Here's how the part is built. I have some questions about the finished solid (model axes, mm). Face numbers are marked on the shaded views. A direction names the side the tool comes from. Round coordinates to 2 decimals unless told otherwise and drop trailing zeros. Order: outer loops, then holes, each group sorted by start corner. A loop starts at its lowest first (then second) coordinate and runs counter-clockwise, first axis right, second up. Notation, with made-up numbers: (-8, 23) -> (12, 23) arc R23 ccw to (12, 49) -> close; hole circle Ø4 at (41, 78.5). An arc over 180 degrees is marked (long way). Answer in a Markdown table with one row per item.
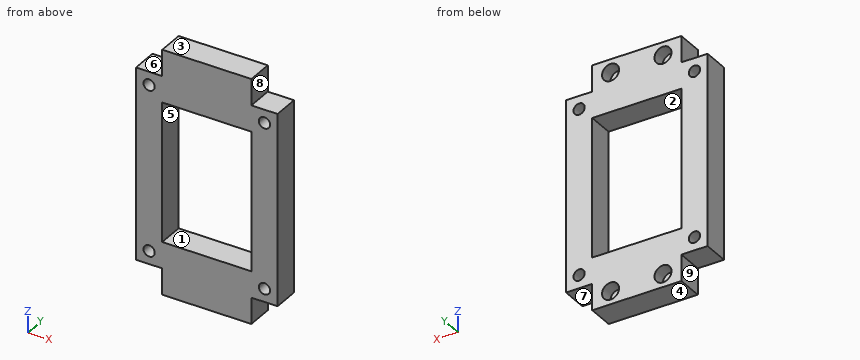
Autodesk Inventor part; units mm, degrees
ref_plane "YZ Plane" through (0, 0, 0) normal (1, 0, 0) x (0, 1, 0)
ref_plane "XZ Plane" through (0, 0, 0) normal (0, 1, 0) x (-1, 0, 0)
ref_plane "XY Plane" through (0, 0, 0) normal (0, 0, 1) x (1, 0, 0)
sketch "Sketch1" plane through (0, 0, 0) normal (0, 1, 0) x (-1, 0, 0)
  line L0 (0, 0) -> (10, 0)
  line L1 (10, 0) -> (10, 10)
  line L2 (10, 10) -> (44, 10)
  line L3 (44, 10) -> (44, 0)
  line L4 (44, 0) -> (54, 0)
  line L5 (54, 0) -> (54, -73)
  line L6 (54, -73) -> (44, -73)
  line L7 (44, -73) -> (44, -83)
  line L8 (44, -83) -> (10, -83)
  line L9 (10, -83) -> (10, -73)
  line L10 (10, -73) -> (0, -73)
  line L11 (0, -73) -> (0, 0)
  dimension "d9" = 73
  dimension "d10" = 54
  dimension "thickness" = 10
  dimension "t" = 10
  dimension "d13" = 10
  dimension "d14" = 10
  dimension "d15" = 10
  dimension "d16" = 10
  dimension "d17" = 10
extrude "Extrusion1" add sketch "Sketch1" along normal blind 10
hole "Hole1" at (-49, 10, -5) direction (0, -1, 0) diameter 4.3 end through all
hole "Hole2" at (-5, 10, -5) direction (0, -1, 0) diameter 4.3 end through all
hole "Hole3" at (-5, 10, -68) direction (0, -1, 0) diameter 4.3 end through all
hole "Hole4" at (-49, 10, -68) direction (0, -1, 0) diameter 4.3 end through all
sketch "Sketch2" plane through (0, 10, 0) normal (0, 1, 0) x (1, 0, 0)
  circle A0 centre (-37, -5) radius 3.25
  circle A1 centre (-17, -5) radius 3.25
  circle A2 centre (-37, 78) radius 3.25
  circle A3 centre (-17, 78) radius 3.25
  line L0 (-44, -10) -> (-10, -10)
  line L1 (-10, 83) -> (-44, 83)
  line L2 (-44, 0) -> (-44, -10)
  line L3 (-10, -10) -> (-10, 0)
  line L4 (-10, 73) -> (-10, 83)
  line L5 (-44, 83) -> (-44, 73)
  point P0 (0, 0)
  dimension "d56" = 6.5
  dimension "d57" = 6.5
  dimension "d58" = 6.5
  dimension "d59" = 6.5
  dimension "d60" = 5
  dimension "d61" = 5
  dimension "d62" = 5
  dimension "d63" = 5
  dimension "d64" = 7
  dimension "d65" = 7
  dimension "d66" = 7
  dimension "d67" = 7
extrude "Extrusion2" cut sketch "Sketch2" against normal blind 5
sketch "Sketch3" plane through (0, 0, 0) normal (0, -1, 0) x (1, 0, 0)
  line L0 (-44, -10) -> (-10, -10)
  line L1 (-10, -10) -> (-10, -63)
  line L2 (-10, -63) -> (-44, -63)
  line L3 (-44, -63) -> (-44, -10)
  line L4 (-10, 10) -> (-44, 10)
  line L5 (-44, -83) -> (-10, -83)
  line L6 (0, -73) -> (0, 0)
  line L7 (-54, 0) -> (-54, -73)
  dimension "d70" = 20
  dimension "d71" = 20
  dimension "d72" = 10
  dimension "d73" = 10
extrude "Extrusion3" cut sketch "Sketch3" against normal blind 10
equation "\"thickness\" = t"
equation "\"d13\" = t"
equation "\"d14\" = t"
equation "\"d15\" = t"
equation "\"d16\" = t"
equation "\"d17\" = t"
equation "\"d18\" = t"
properties part number "backFrame"
1. For the marked faces 5, 6, 7, 8 and 9, which set-ups out of +Z, -Z, +X, -X, +Y, -Y let a thin tool reach every point of the face, with its end or its side?
Numbers:
| item | result |
|---|---|
| face 5 | +Y, -Y |
| face 6 | +Z, -X, +Y, -Y |
| face 7 | -Z, +X, +Y, -Y |
| face 8 | +Z, +X, +Y, -Y |
| face 9 | -Z, -X, +Y, -Y |
2. Suppose I cut it at C-C on y = 8. State how many separate pieces and enclosed holes the cut face has, then the cut area to 3 significant figures.
Numbers:
| item | result |
|---|---|
| separate pieces | 1 |
| enclosed holes | 9 |
| area | 2,630 mm2 |
3. Suppose I cut it at D-D on z = -25. Write out the boundary of the cut face in (x, y), then the cut area to 3 significant figures.
Numbers:
| item | result |
|---|---|
| outline | (-54, 0) -> (-44, 0) -> (-44, 10) -> (-54, 10) -> close; (-10, 0) -> (0, 0) -> (0, 10) -> (-10, 10) -> close |
| area | 200 mm2 |
4. For pin 1 Ø5 at (x, y) = (-4.5, 7) entering from -Z; pin 2 Ø3 at (y, z) = (3, -79.5) entering from +X; pin 3 Ø3 at (x, z) = (-37.5, 5) entering from +Y, each with a flat end and sliding along its axis, tell me the tip position at first contact or that it passes through.
Numbers:
| item | result |
|---|---|
| pin 1 | stops at z = -73 |
| pin 2 | stops at x = -10 |
| pin 3 | stops at y = 5 |
5. We'd pull the mould along Z, two halves only. Please class the marked faces 1, 2, 3 and 4: released by +Z, released by -Z, zero draft, split by the parting line, or undercut.
Numbers:
| item | result |
|---|---|
| face 1 | undercut |
| face 2 | undercut |
| face 3 | released by +Z |
| face 4 | released by -Z |
6. Suppose I cut it at A-A on x = -28.5. Write out the boundary of the cut face in (y, z), then the cut area to 3 significant figures.
Numbers:
| item | result |
|---|---|
| outline | (0, -83) -> (10, -83) -> (10, -63) -> (0, -63) -> close; (0, -10) -> (10, -10) -> (10, 10) -> (0, 10) -> close |
| area | 400 mm2 |
7. Suppose I cut it at B-B on z = -5. Write out the boundary of the cut face in (x, y), then the cut area to 3 significant figures.
Numbers:
| item | result |
|---|---|
| outline | (-54, 0) -> (-51.15, 0) -> (-51.15, 10) -> (-54, 10) -> close; (-46.85, 0) -> (-7.15, 0) -> (-7.15, 10) -> (-46.85, 10) -> close; (-2.85, 0) -> (0, 0) -> (0, 10) -> (-2.85, 10) -> close |
| area | 454 mm2 |
8. Please list where these lines run through material, in increasing order: line 1 along Z through (x, y) = (-5, 5.25); line 2 along X through (y, z) = (7.5, -5); line 3 along X through (y, z) = (9.05, -78).
Numbers:
| item | result |
|---|---|
| line 1 | z = -73 to -70.15, -65.85 to -7.15, -2.85 to 0 |
| line 2 | x = -54 to -51.15, -46.85 to -7.15, -2.85 to 0 |
| line 3 | x = -44 to -40.25, -33.75 to -20.25, -13.75 to -10 |
